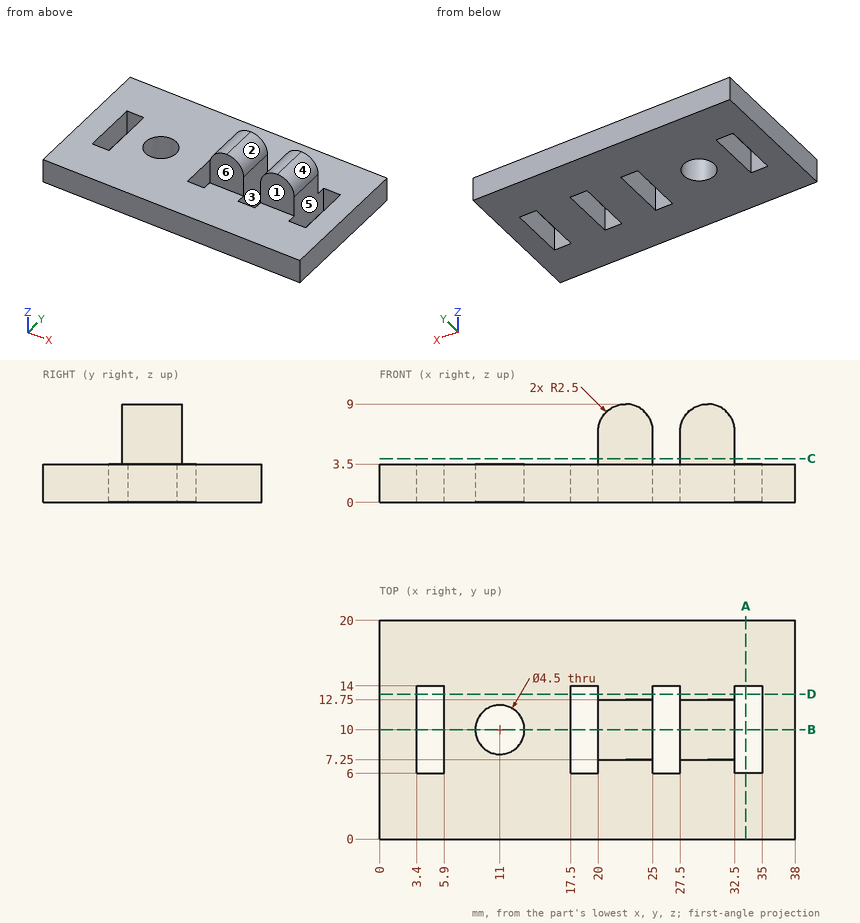
Input: dimensioned drawing with shaded views. Units: mm. Origin: part minimum x, y, z. A direction names the side the tool comes from. Round coordinates to 2 decimals unless told otherwise and drop trailing zeros. Write each loop counter-clockwise with the first axis right and the second up, starting at its lowest first coordinate (ties: lowest second). Pieces come first, ordered by that corner, then holes. Notation, with made-up numbers: (55, 48.5) - (70, 48.5) arc R17 ccw to (70, 56.5) - close; hole circle Ø2 at (71.5, -1). An arc over 180 degrees is marked (long way). Write item = value, one per line.
(1) Contact query for flat-ended pins moving along their axis: pin 1 Ø5 at (x, y) = (34, 13.5) entering from -Z; pin 2 Ø2.5 at (x, z) = (21.5, 5) entering from +Y; pin 3 Ø1 at (x, y) = (14, 11.5) entering from +Z; pin 4 Ø1.5 at (x, z) = (23.5, 7.5) entering from -Y. Output: stop coordinate, or through.
Geometry check:
pin_1 = 0
pin_2 = 12.75
pin_3 = 3.5
pin_4 = 7.25
(2) Pull-direction query (Y, two-part tool) for the marked faces 4, 5 and 6; classes: +Y half, -Y half, draft (parallel to the pull), parting line (faces both ways), or undercut.
Geometry check:
face_4 = draft
face_5 = undercut
face_6 = -Y half
(3) Section query B-B on y = 10. State how many separate pieces and enclosed holes the cut face has, then the cut area to 3 significant figures.
Geometry check:
separate_pieces = 6
enclosed_holes = 0
area = 132 mm^2
(4) Section query D-D on y = 13.25. Output: boundary loops of the cut face in (x, z).
Geometry check:
outline = (0, 0) - (3.4, 0) - (3.4, 3.5) - (0, 3.5) - close; (5.9, 0) - (17.5, 0) - (17.5, 3.5) - (5.9, 3.5) - close; (20, 0) - (25, 0) - (25, 3.5) - (20, 3.5) - close; (27.5, 0) - (32.5, 0) - (32.5, 3.5) - (27.5, 3.5) - close; (35, 0) - (38, 0) - (38, 3.5) - (35, 3.5) - close
(5) Section query A-A on x = 33.5. Output: boundary loops of the cut face in (y, z), then the cut area to 3 significant figures.
Geometry check:
outline = (0, 0) - (6, 0) - (6, 3.5) - (0, 3.5) - close; (14, 0) - (20, 0) - (20, 3.5) - (14, 3.5) - close
area = 42.0 mm^2
(6) Section query C-C on z = 4. Output: boundary loops of the cut face in (x, y).
Geometry check:
outline = (20, 7.25) - (25, 7.25) - (25, 12.75) - (20, 12.75) - close; (27.5, 7.25) - (32.5, 7.25) - (32.5, 12.75) - (27.5, 12.75) - close
(7) Material intervals for probe 1 along Y at (x, z) = (11, 1.95); probe 2 along X at (y, z) = (9.5, 2); probe 3 along Z at (x, y) = (9, 1), sorted ascending.
Geometry check:
probe_1 = 0 to 7.75, 12.25 to 20
probe_2 = 0 to 3.4, 5.9 to 8.81, 13.19 to 17.5, 20 to 25, 27.5 to 32.5, 35 to 38
probe_3 = 0 to 3.5
(8) Access query for the marked faces 1, 2 and 3. Directions: +Z, -Z, +X, -X, +Y, -Y. A direction counts if a zero-diameter tool reaches every point of the face in a straight line with its end or side. Return the directions, or none.
Geometry check:
face_1 = +Z, +X, -X, -Y
face_2 = +Z, +Y, -Y
face_3 = +Z, -Z
